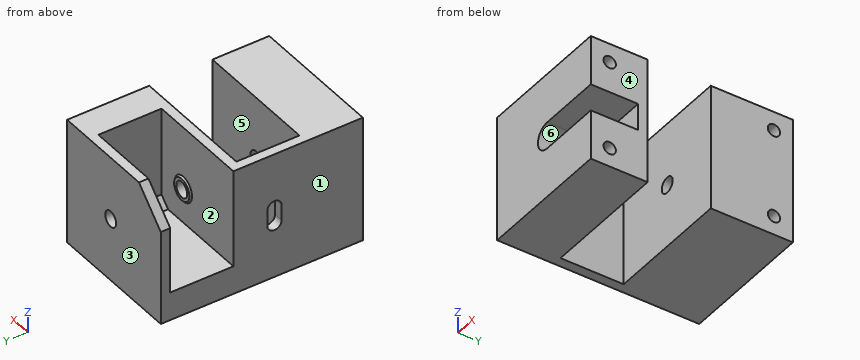
```python
from build123d import *

# Parameters (mm, degrees)
BOSS_EXTRUDE1_DEPTH     = 40
CUT_EXTRUDE1_DEPTH      = 70.94998213
CUT_EXTRUDE1_DEPTH_BACK = 70.94998213
SKETCH3_R               = 2.5
CUT_EXTRUDE2_DEPTH      = 15
SKETCH5_R               = 3.5
SKETCH5_R_2             = 2.5
BOSS_EXTRUDE2_DEPTH     = 0.5
BOSS_EXTRUDE3_START     = 0.5
SKETCH6_R               = 3.5
SKETCH6_R_2             = 2.5
BOSS_EXTRUDE3_DEPTH     = 0.5
CHAMFER1_SIZE           = 0.5
CUT_EXTRUDE3_DEPTH      = 4.159338157
SKETCH9_W               = 43
SKETCH9_H               = 23
BOSS_EXTRUDE4_DEPTH     = 9
CHAMFER2_SIZE           = 3
SKETCH8_R               = 1.95
CUT_EXTRUDE4_DEPTH      = 9
CHAMFER5_SIZE           = 10


with BuildPart() as part:
    # Sketch1 → Boss-Extrude1 (new body)
    with BuildSketch(Plane.XY):
        Polygon((0, 0), (-40, 0), (-40, 20), (0, 20), (0, 46), (-43, 46), (-43, 43), (-10, 43), (-10, 23), (-43, 23), (-43, -18), (0, -18), align=None)
    extrude(amount=BOSS_EXTRUDE1_DEPTH)

    # Sketch3 → Cut-Extrude1 (cut, two sides: drawn at the far end of the back side and taken through both)
    with BuildSketch(Plane(origin=(0, 20, 0), x_dir=(-1, 0, 0), z_dir=(0, -1, 0)).offset(-CUT_EXTRUDE1_DEPTH_BACK)):
        with Locations(Location((20, -20, 0), (0, 0, 180))):
            Circle(SKETCH3_R)
    extrude(amount=CUT_EXTRUDE1_DEPTH + CUT_EXTRUDE1_DEPTH_BACK, mode=Mode.SUBTRACT)

    # Sketch4 → Cut-Extrude2 (cut)
    with BuildSketch(Plane(origin=(0, -18, 0), x_dir=(-1, 0, 0), z_dir=(0, -1, 0))):
        with BuildLine():
            Line((20, -24.25), (0, -24.25))
            Line((0, -24.25), (0, -15.75))
            Line((0, -15.75), (20, -15.75))
            ThreePointArc((20, -15.75), (24.25, -20), (20, -24.25))
        make_face()
    extrude(amount=-CUT_EXTRUDE2_DEPTH, mode=Mode.SUBTRACT)

    # Sketch5 → Boss-Extrude2 (add)
    with BuildSketch(Plane(origin=(0, 23, 0), x_dir=(1, 0, 0), z_dir=(0, 1, 0))):
        with Locations(Location((-20, -20, 0), (0, 0, 90))):
            Circle(SKETCH5_R)
        with Locations((-20, -20)):
            Circle(SKETCH5_R_2, mode=Mode.SUBTRACT)
    extrude(amount=BOSS_EXTRUDE2_DEPTH)

    # Sketch6 → Boss-Extrude3 (add)
    with BuildSketch(Plane(origin=(0, 43, 0), x_dir=(-1, 0, 0), z_dir=(0, -1, 0)).offset(BOSS_EXTRUDE3_START)):
        with Locations(Location((20, -20, 0), (0, 0, 90))):
            Circle(SKETCH6_R)
        with Locations(Location((20, -20, 0), (0, 0, 180))):
            Circle(SKETCH6_R_2, mode=Mode.SUBTRACT)
    extrude(amount=-BOSS_EXTRUDE3_DEPTH)

    # Chamfer1
    chamfer1_edges = [part.edges().sort_by_distance(p)[0] for p in [
        (-20, 23, 23.5),
        (-20, 43, 23.5),
    ]]
    chamfer(chamfer1_edges, length=CHAMFER1_SIZE - 0.0001)  # a hair under: the kernel refuses the full size

    # Sketch7 → Cut-Extrude3 (cut)
    with BuildSketch(Plane(origin=(-40, 0, 0), x_dir=(0, 0, -1), z_dir=(1, 0, 0))):
        with BuildLine():
            Line((-22.5, 12.25), (-17.5, 12.25))
            ThreePointArc((-17.5, 12.25), (-15.25, 10), (-17.5, 7.75))
            Line((-17.5, 7.75), (-22.5, 7.75))
            ThreePointArc((-22.5, 7.75), (-24.75, 10), (-22.5, 12.25))
        make_face()
    extrude(amount=-CUT_EXTRUDE3_DEPTH, mode=Mode.SUBTRACT)

    # Sketch9 → Boss-Extrude4 (add)
    with BuildSketch(Plane(origin=(0, 0, 0), x_dir=(-1, 0, 0), z_dir=(0, 0, -1))):
        with Locations((21.5, 34.5)):
            Rectangle(SKETCH9_W, SKETCH9_H)
    extrude(amount=-BOSS_EXTRUDE4_DEPTH)

    # Chamfer2
    chamfer2_edges = [part.edges().sort_by_distance(p)[0] for p in [
        (-10, 33, 9),
    ]]
    chamfer(chamfer2_edges, length=CHAMFER2_SIZE)

    # Sketch8 → Cut-Extrude4 (cut)
    with BuildSketch(Plane(origin=(0, 0, 0), x_dir=(0, 0, -1), z_dir=(1, 0, 0))):
        with Locations(Location((-34, 40, 0), (0, 0, 90))):
            Circle(SKETCH8_R)
        with Locations(Location((-6, 40, 0), (0, 0, 90))):
            Circle(SKETCH8_R)
        with Locations(Location((-34, -12, 0), (0, 0, 90))):
            Circle(SKETCH8_R)
        with Locations(Location((-6, -12, 0), (0, 0, 90))):
            Circle(SKETCH8_R)
    extrude(amount=-CUT_EXTRUDE4_DEPTH, mode=Mode.SUBTRACT)

    # Chamfer5
    chamfer5_edges = [part.edges().sort_by_distance(p)[0] for p in [
        (-43, 44.5, 40),
    ]]
    chamfer(chamfer5_edges, length=CHAMFER5_SIZE)


solid = part.part
```
For this review, take the finished solid that the model builds, in its own axes (mm). Face numbers are marked on the shaded views. A direction names the side the tool comes from. Coordinates: 2 decimals unless noted, no trailing zeros. Write each loop counter-clockwise with the first axis right and the second up, starting at its lowest first coordinate (ties: lowest second). Pieces come first, ordered by that corner, then holes.
(1) Add section A-A on x = -12. Give the boundary of the cut face in (y, z).
(2) The part is to be moulded in two halves that separate along Y. For the marked faces 1, 2 and 3, say which applies: +Y half, -Y half, draft (parallel to the pull), parting line (faces both ways), or undercut.
(3) Add section B-B on y = 10. Give the boundary of the cut face in (x, z).
(4) For pin 1 Ø10 at (y, z) = (37.5, 33) entering from -X; pin 2 Ø3 at (y, z) = (13.5, 15.5) entering from +X; pin 3 Ø8 at (x, z) = (-20, 20) entering from -Y, all flat-tipped, find the tip position at first contact; note any pin that passes through.
(5) Tool access review of the marked faces 4, 5 and 6: name each direction out of +Z, -Z, +X, -X, +Y, -Y from which nothing blocks a thin tool from reaching the whole face with its end or side.
(6) Wall thickness on probe 1 along Z at (x, y) = (-6, 40); probe 2 along Y at (x, z) = (-11, 32); probe 3 along Y at (x, z) = (-2.5, 9.5): over which ranges is each line inside the solid? List them lowest first.
(7) Add section C-C on z = 27. Give the boundary of the cut face in (x, y).
(8) Add section D-D on x = -34. Give the boundary of the cut face in (y, z), then the cut area to 3 significant figures.
Answer sheet:
1. outline: (-18, 0) - (0, 0) - (0, 40) - (-18, 40) - (-18, 24.25) - (-3, 24.25) - (-3, 15.75) - (-18, 15.75) - close; (20, 0) - (46, 0) - (46, 40) - (43, 40) - (43, 10) - (23, 10) - (23, 40) - (20, 40) - close
2. face 1: draft
2. face 2: undercut
2. face 3: +Y half
3. outline: (-43, 0) - (-40, 0) - (-40, 15.25) - (-43, 15.25) - close; (-43, 24.75) - (-40, 24.75) - (-40, 40) - (-43, 40) - close
4. pin 1: stops at x = -10
4. pin 2: stops at x = -40
4. pin 3: stops at y = -3
5. face 4: +Z, -Z, +X, +Y, -Y
5. face 5: +Z, -Z, +X
5. face 6: +X, -Y
6. probe 1: z = 0 to 4.05, 7.95 to 32.05, 35.95 to 40
6. probe 2: y = -18 to 0, 20 to 23, 43 to 46
6. probe 3: y = -18 to 0, 20 to 46
7. outline: (-43, -18) - (0, -18) - (0, 0) - (-40, 0) - (-40, 20) - (0, 20) - (0, 46) - (-43, 46) - (-43, 43) - (-10, 43) - (-10, 23) - (-43, 23) - close
8. outline: (-18, 0) - (0, 0) - (0, 40) - (-18, 40) - close; (20, 0) - (46, 0) - (46, 39) - (43, 39) - (43, 9) - (23, 9) - (23, 40) - (20, 40) - close
8. area: 1,140 mm2
